Source: CAD feature listing. Evaluate the final solid. Frame: model axes, mm. Face numbers are marked on the shaded views. A direction names the side the tool comes from. Give positions to 0.01 mm unless a question says otherwise; leave off trailing zeros. Order: outer loops, then holes, each group sorted by start corner. A loop starts at its lowest first (then second) coordinate and runs counter-clockwise, first axis right, second up. Notation, with made-up numbers: (65, -24.75) - (107, -24.75) arc R15 cw to (107, -16.75) - close; hole circle Ø9 at (56.5, 84). An arc over 180 degrees is marked (long way). Write each question's results on one line, items separated by ' | '. Start each with the question number.
Item 1: Section D-D on y = -1. Output: boundary loops of the cut face in (x, z) (3 decimals).
Item 2: Section B-B on x = -25. Output: boundary loops of the cut face in (y, z) (3 decimals).
Item 3: Section C-C on x = 13. Output: boundary loops of the cut face in (y, z) (3 decimals).
Item 4: Line query: line 1 along Y through (x, z) = (-27, 46.5) (3 decimals); line 2 along Z through (x, y) = (11.5, 4); line 3 along Z through (x, y) = (-3, -6.5). Output: solid intervals per line, ascending.
Item 5: Set-up query: the marked faces 1, 2, 3 and 4. Return all of +Z, -Z, +X, -X, +Y, -Y with unobstructed straight access to the full face (end or side cutting, diameter ignored); none if empty.
Item 6: Section A-A on z = 10.5. Output: boundary loops of the cut face in (x, y) (3 decimals), and give its area (3 significant figures).
Item 7: Contact query for flat-ended pins moving along their axis: pin 1 Ø4 at (y, z) = (-4, 44.5) entering from -X; pin 2 Ø6 at (y, z) = (5.5, 26) entering from +X (3 decimals); pin 3 Ø5 at (x, z) = (-9.5, -15) entering from -Y; pin 4 Ø3 at (y, z) = (-0.5, -16.5) entering from -X. Output: stop coordinate, or through.
Item 8: Mould query, pull axis Y, two halves, no side actions, for the marked faces 5, 6 and 7. Classes: released by +Y, released by -Y, zero draft, split by the parting line, or undercut.
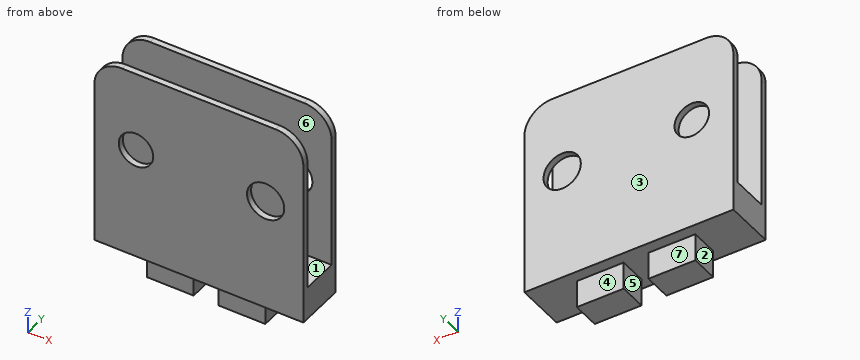
```python
from build123d import *

# Parameters (mm, degrees)
SKETCH1_W           = 75.79
SKETCH1_H           = 18
BOSS_EXTRUDE1_DEPTH = 60
SKETCH2_W           = 75.79
SKETCH2_H           = 13.45
CUT_EXTRUDE1_DEPTH  = 58
SKETCH7_R           = 6.260869565
SKETCH7_R_2         = 6.760869565
CUT_EXTRUDE3_DEPTH  = 74.212232755
SKETCH6_W           = 75.79
SKETCH6_H           = 18
BOSS_EXTRUDE2_DEPTH = 10
SKETCH8_W           = 17
SKETCH8_H           = 10
BOSS_EXTRUDE3_DEPTH = 10
FILLET1_R           = 10


with BuildPart() as part:
    # Sketch1 → Boss-Extrude1 (new body)
    with BuildSketch(Plane.XY):
        Rectangle(SKETCH1_W, SKETCH1_H)
    extrude(amount=BOSS_EXTRUDE1_DEPTH)

    # Sketch2 → Cut-Extrude1 (cut)
    with BuildSketch(Plane.XY.offset(60)):
        Rectangle(SKETCH2_W, SKETCH2_H)
    extrude(amount=-CUT_EXTRUDE1_DEPTH, mode=Mode.SUBTRACT)

    # Sketch7 → Cut-Extrude3 (cut, through all)
    with BuildSketch(Plane(origin=(0, 9, 0), x_dir=(1, 0, 0), z_dir=(0, 1, 0))):
        with Locations(Location((-22.807801707, -30.844118328, 0), (0, 0, 270))):
            Circle(SKETCH7_R)
        with Locations(Location((24.199095104, -30.844118328, 0), (0, 0, 270))):
            Circle(SKETCH7_R_2)
    extrude(amount=-CUT_EXTRUDE3_DEPTH, mode=Mode.SUBTRACT)

    # Sketch6 → Boss-Extrude2 (add)
    with BuildSketch(Plane(origin=(0, 0, 0), x_dir=(-1, 0, 0), z_dir=(0, 0, -1))):
        Rectangle(SKETCH6_W, SKETCH6_H)
    extrude(amount=BOSS_EXTRUDE2_DEPTH)

    # Sketch8 → Boss-Extrude3 (add)
    with BuildSketch(Plane(origin=(0, 0, -10), x_dir=(-1, 0, 0), z_dir=(0, 0, -1))):
        with Locations((-13, 0)):
            Rectangle(SKETCH8_W, SKETCH8_H)
        with Locations((13, 0)):
            Rectangle(SKETCH8_W, SKETCH8_H)
    extrude(amount=BOSS_EXTRUDE3_DEPTH)

    # Fillet1
    fillet1_edges = [part.edges().sort_by_distance(p)[0] for p in [
        (-37.895, 7.8625, 60),
        (37.895, 7.8625, 60),
        (-37.895, -7.8625, 60),
        (37.895, -7.8625, 60),
    ]]
    fillet(fillet1_edges, radius=FILLET1_R)


solid = part.part
```
Evaluation:
1) outline: (-37.895, -10) - (-21.5, -10) - (-21.5, -20) - (-4.5, -20) - (-4.5, -10) - (4.5, -10) - (4.5, -20) - (21.5, -20) - (21.5, -10) - (37.895, -10) - (37.895, 2) - (-37.895, 2) - close
2) outline: (-9, -10) - (9, -10) - (9, 24.98) - (6.725, 24.98) - (6.725, 2) - (-6.725, 2) - (-6.725, 24.98) - (-9, 24.98) - close; (-9, 36.709) - (-6.725, 36.709) - (-6.725, 60) - (-9, 60) - close; (6.725, 36.709) - (9, 36.709) - (9, 60) - (6.725, 60) - close
3) outline: (-9, -10) - (-5, -10) - (-5, -20) - (5, -20) - (5, -10) - (9, -10) - (9, 60) - (6.725, 60) - (6.725, 2) - (-6.725, 2) - (-6.725, 60) - (-9, 60) - close
4) line 1: y = -9 to -6.725, 6.725 to 9 | line 2: z = -20 to 2 | line 3: z = -10 to 2
5) face 1: +Z, +X, -X | face 2: -Z, -X, +Y, -Y | face 3: +Z, -Z, +X, -X, +Y | face 4: -Z, +X, -X, +Y
6) outline: (-37.895, -9) - (37.895, -9) - (37.895, -6.725) - (-37.895, -6.725) - close; (-37.895, 6.725) - (37.895, 6.725) - (37.895, 9) - (-37.895, 9) - close | area: 345 mm^2
7) pin 1: passes through | pin 2: stops at x = 37.895 | pin 3: stops at y = -5 | pin 4: stops at x = -21.5
8) face 5: zero draft | face 6: undercut | face 7: released by +Y
